```python
from build123d import *
from build123d.topology import SkipClean

# Parameters (mm, degrees)
SKETCH1_R           = 6.45
BOSS_EXTRUDE1_DEPTH = 15
SKETCH2_W           = 5
SKETCH2_H           = 3
CUT_EXTRUDE3_DEPTH  = 5
CUT_EXTRUDE4_START  = -40
SKETCH4_R           = 1.5
CUT_EXTRUDE4_DEPTH  = 63
SKETCH5_R           = 3
CUT_EXTRUDE5_DEPTH  = 4
CUT_EXTRUDE6_START  = -80
CUT_EXTRUDE6_DEPTH  = 80


with BuildPart() as part:
    # Sketch1 → Boss-Extrude1 (new body)
    with BuildSketch(Plane.XY):
        with BuildLine():
            Line((0, 23), (0, 37))
            Line((0, 37), (12.859510911, 37))
            Line((12.859510911, 37), (12.859510911, 27))
            ThreePointArc((12.859510911, 27), (20.383390121, 21.88342816), (26.020458433, 14.741192754))
            Line((26.020458433, 14.741192754), (28.050458433, 14.741192754))
            Line((28.050458433, 14.741192754), (28.050458433, 9.460443964))
            ThreePointArc((28.050458433, 9.460443964), (34.500458433, 11.45), (40.950458433, 9.460443964))
            Line((40.950458433, 9.460443964), (40.950458433, 32.5))
            Line((40.950458433, 32.5), (50.950458433, 32.5))
            Line((50.950458433, 32.5), (50.950458433, -32.5))
            Line((50.950458433, -32.5), (40.950458433, -32.5))
            Line((40.950458433, -32.5), (40.950458433, -9.460443964))
            ThreePointArc((40.950458433, -9.460443964), (34.500458433, -11.45), (28.050458433, -9.460443964))
            Line((28.050458433, -9.460443964), (28.050458433, -14.741192754))
            Line((28.050458433, -14.741192754), (26.020458433, -14.741192754))
            ThreePointArc((26.020458433, -14.741192754), (20.383390121, -21.88342816), (12.859510911, -27))
            Line((12.859510911, -27), (12.859510911, -37))
            Line((12.859510911, -37), (0, -37))
            Line((0, -37), (0, -23))
            ThreePointArc((0, -23), (23, 0), (0, 23))
        make_face()
        with Locations(Location((34.500458433, 0, 0), (0, 0, 180))):
            Circle(SKETCH1_R, mode=Mode.SUBTRACT)
    boss_extrude1 = extrude(amount=BOSS_EXTRUDE1_DEPTH)

    # Sketch2 → Cut-Revolve1 (revolve, cut)
    with BuildSketch(Plane.ZY):
        with Locations((7.5, 24.5)):
            Rectangle(SKETCH2_W, SKETCH2_H)
    cut_revolve1 = revolve(axis=Axis((0, 0, 15), (0, 0, -1)), mode=Mode.SUBTRACT)

    # Sketch3 → Cut-Extrude3 (cut)
    with BuildSketch(Plane(origin=(50.950458433, 0, 0), x_dir=(0, 0, -1), z_dir=(1, 0, 0))):
        with BuildLine():
            Line((-12.5, -25), (-12.5, 25))
            ThreePointArc((-12.5, 25), (-7.5, 30), (-2.5, 25))
            Line((-2.5, 25), (-2.5, -25))
            ThreePointArc((-2.5, -25), (-7.5, -30), (-12.5, -25))
        make_face()
    extrude(amount=-CUT_EXTRUDE3_DEPTH, mode=Mode.SUBTRACT)

    # Sketch4 → Cut-Extrude4 (cut)
    with BuildSketch(Plane(origin=(12.859510911, 0, 0), x_dir=(0, 0, -1), z_dir=(1, 0, 0)).offset(CUT_EXTRUDE4_START)):
        with Locations((-7.333431897, 32)):
            Circle(SKETCH4_R)
        with Locations((-7.333431897, -32)):
            Circle(SKETCH4_R)
    cut_extrude4 = extrude(amount=CUT_EXTRUDE4_DEPTH, mode=Mode.SUBTRACT)

    # Sketch5 → Cut-Extrude5 (cut)
    with BuildSketch(Plane(origin=(12.859510911, 0, 0), x_dir=(0, 0, -1), z_dir=(1, 0, 0))):
        with Locations((-7.5, 32)):
            Circle(SKETCH5_R)
        with Locations(Location((-7.5, -32, 0), (0, 0, 180))):
            Circle(SKETCH5_R)
    cut_extrude5 = extrude(amount=-CUT_EXTRUDE5_DEPTH, mode=Mode.SUBTRACT)

    # Mirror1: Boss-Extrude1, Cut-Revolve1, Cut-Extrude4, Cut-Extrude5 across plane
    add(boss_extrude1.mirror(Plane.ZY))
    add(cut_revolve1.mirror(Plane.ZY), mode=Mode.SUBTRACT)
    add(cut_extrude4.mirror(Plane.ZY), mode=Mode.SUBTRACT)
    add(cut_extrude5.mirror(Plane.ZY), mode=Mode.SUBTRACT)

    # Sketch6 → Cut-Extrude6 (cut)
    with SkipClean():  # the faces are left unmerged after this step: merging them gives an invalid solid
        with BuildSketch(Plane.XY.offset(15).offset(CUT_EXTRUDE6_START)):
            with BuildLine():
                Line((-40.950458433, 9.460443964), (-40.950458433, 38.741811421))
                Line((-40.950458433, 38.741811421), (-62.772471418, 38.741811421))
                Line((-62.772471418, 38.741811421), (-62.772471418, -39.471412389))
                Line((-62.772471418, -39.471412389), (-40.950458433, -39.471412389))
                Line((-40.950458433, -39.471412389), (-40.950458433, -9.460443964))
                ThreePointArc((-40.950458433, -9.460443964), (-45.950458433, 0), (-40.950458433, 9.460443964))
            make_face()
        extrude(amount=CUT_EXTRUDE6_DEPTH, mode=Mode.SUBTRACT)


solid = part.part
```
Source: CAD feature listing. Evaluate the final solid. Frame: model axes, mm. A direction names the side the tool comes from. Round coordinates to 2 decimals unless told otherwise and drop trailing zeros. Loops run counter-clockwise (first coordinate to the right, second up) from the corner with the lowest first, then second, coordinate; pieces in that order, holes last.
1. Section query B-B on x = 14.5. Output: boundary loops of the cut face in (y, z).
2. Access query for faces 4 (the flat face through (-27, -14.741, 7)), 5 (the flat face through (40.95, 21, 7)), 6 (the cylindrical face through (20.477, -21.796, 7.395)), 7 (the flat face through (48, 0, 2.5)), 8 (the flat face through (-8.86, 32, 9)). Directions: +Z, -Z, +X, -X, +Y, -Y. A direction counts if a zero-diameter tool reaches every point of the face in a straight line with its end or side. Return the directions, or none.
3. Section query A-A on y = 0. Output: boundary loops of the cut face in (x, z), and give its area (3 significant figures).
4. Mould query, pull axis Z, two halves, no side actions, for faces 1 (the flat face through (0, 37, 7)), 2 (the flat face through (8.86, -31, 9)), 3 (the flat face through (25, 1, 15)). Classes: released by +Z, released by -Z, zero draft, split by the parting line, or undercut.
5. Contact query for flat-ended pins moving along their axis: pin 1 (2.5 mm diameter, centred on y = -13, z = 8, fed in from -X); pin 2 (8 mm diameter, centred on y = -21, z = 4.5, fed in from +X); pin 3 (4 mm diameter, centred on x = 37.5, z = 6.5, fed in from +Y); pin 4 (1.8 mm diameter, centred on y = 32, z = 7.33, fed in from -X). Output: stop coordinate, or through.
6. Ray query, L1, parallel to X at y = 30, z = 6; L2, parallel to Y at x = 11.7, z = 7.5; L3, parallel to X at y = 12.5, z = 13.75. Return the intervals inside material, ascending.
7. Section query D-D on y = -21. Output: boundary loops of the cut face in (x, z).
8. Section query C-C on z = 14. Give the number of separate pieces and of enclosed holes in the cut face, and give its area (3 significant figures).
Answers below:
1. outline: (-26.16, 0) - (-17.85, 0) - (-17.85, 5) - (-21.58, 5) - (-21.58, 10) - (-17.85, 10) - (-17.85, 15) - (-26.16, 15) - close; (17.85, 0) - (26.16, 0) - (26.16, 15) - (17.85, 15) - (17.85, 10) - (21.58, 10) - (21.58, 5) - (17.85, 5) - close
2. face 4: +Z, -Z, -X, -Y
2. face 5: +Z, -Z, +Y
2. face 6: +Z, -Z, -Y
2. face 7: +X
2. face 8: -X
3. outline: (-45.95, 0) - (-40.95, 0) - (-40.95, 15) - (-45.95, 15) - close; (-28.05, 0) - (-23, 0) - (-23, 5) - (-26, 5) - (-26, 10) - (-23, 10) - (-23, 15) - (-28.05, 15) - close; (23, 0) - (28.05, 0) - (28.05, 15) - (23, 15) - (23, 10) - (26, 10) - (26, 5) - (23, 5) - close; (40.95, 0) - (50.95, 0) - (50.95, 2.5) - (45.95, 2.5) - (45.95, 12.5) - (50.95, 12.5) - (50.95, 15) - (40.95, 15) - close
3. area: 297 mm2
4. face 1: zero draft
4. face 2: undercut
4. face 3: released by +Z
5. pin 1: stops at x = -28.05
5. pin 2: stops at x = 50.95
5. pin 3: stops at y = 11.41
5. pin 4: stops at x = 40.95
6. L1: x = -8.86 to 8.86, 40.95 to 50.95
6. L2: y = -37 to -35, -29 to -23.22, 23.22 to 29, 35 to 37
6. L3: x = -28.05 to -19.31, 19.31 to 28.05, 40.95 to 50.95
7. outline: (-21.29, 0) - (-9.38, 0) - (-9.38, 5) - (-15.33, 5) - (-15.33, 10) - (-9.38, 10) - (-9.38, 15) - (-21.29, 15) - close; (9.38, 0) - (21.29, 0) - (21.29, 15) - (9.38, 15) - (9.38, 10) - (15.33, 10) - (15.33, 5) - (9.38, 5) - close; (40.95, 0) - (50.95, 0) - (50.95, 2.5) - (45.95, 2.5) - (45.95, 12.5) - (50.95, 12.5) - (50.95, 15) - (40.95, 15) - close
8. separate pieces: 1
8. enclosed holes: 3
8. area: 2,540 mm2
